Part model, mm, in its own coordinate system. A direction names the side the tool comes from. Give positions to 0.01 mm unless a question says otherwise; leave off trailing zeros. Loops run counter-clockwise (first coordinate to the right, second up) from the corner with the lowest first, then second, coordinate; pieces in that order, holes last. Notation, with made-up numbers: M -9,38 L 47,38 A33 cw 47,74 Z; hole C -12.5,30 d2. An arc over 180 degrees is marked long. Answer in a Markdown table with one row per item.
from build123d import *

# Parameters (mm, degrees)
F1_DEPTH = 4


with BuildPart() as f1:
    # F0 (on Front) → F1 (new body, symmetric)
    with BuildSketch(Plane.XZ):
        with BuildLine():
            ThreePointArc((111.130167, 15.609894), (95.033027, 8.473776), (77.595073, 6.0325))
            Line((77.595073, 6.0325), (-77.595073, 6.0325))
            ThreePointArc((-77.595073, 6.0325), (-95.033027, 8.473776), (-111.130167, 15.609894))
            ThreePointArc((-111.130167, 15.609894), (-161.194556, 29.17665), (-210.450019, 12.91629))
            ThreePointArc((-210.450019, 12.91629), (-213.914336, 11.208725), (-217.731712, 10.621431))
            Line((-217.731712, 10.621431), (-225.425, 10.621431))
            Line((-225.425, 10.621431), (-225.425, 0))
            Line((-225.425, 0), (-225.191568, 0))
            Line((-225.191568, 0), (-217.639167, 0))
            ThreePointArc((-217.639167, 0), (-213.437314, 0.715242), (-209.708742, 2.780405))
            ThreePointArc((-209.708742, 2.780405), (-161.129499, 20.611828), (-111.59344, 5.64248))
            ThreePointArc((-111.59344, 5.64248), (-94.152949, -3.043403), (-74.899881, -6.0325))
            Line((-74.899881, -6.0325), (74.899881, -6.0325))
            ThreePointArc((74.899881, -6.0325), (94.152949, -3.043403), (111.59344, 5.64248))
            ThreePointArc((111.59344, 5.64248), (161.129499, 20.611828), (209.708742, 2.780405))
            ThreePointArc((209.708742, 2.780405), (213.437314, 0.715242), (217.639167, 0))
            Line((217.639167, 0), (225.191568, 0))
            Line((225.191568, 0), (225.425, 0))
            Line((225.425, 0), (225.425, 10.621431))
            Line((225.425, 10.621431), (217.731712, 10.621431))
            ThreePointArc((217.731712, 10.621431), (213.914336, 11.208725), (210.450019, 12.91629))
            ThreePointArc((210.450019, 12.91629), (161.194556, 29.17665), (111.130167, 15.609894))
        make_face()
    extrude(amount=F1_DEPTH, both=True)


solid = f1.part
(1) Which spindle directions (+Z, -Z, +X, -X, +Y, -Y) get a long thin tool onto all of the face, cutting with end or side? Do faces 5 (the face through (-94.795, -0.056, 8.406)), 6 (the face through (221, 0, 0)), 7 (the face through (-222, 0, 0)), 8 (the face through (-213.494, -0.056, 0.696)), 9 (the face through (222, 0, 10.621)). Say none if no direction does.
Recorded:
| item | result |
|---|---|
| face 5 | +Z, +Y, -Y |
| face 6 | -Z, +X, +Y, -Y |
| face 7 | -Z, -X, +Y, -Y |
| face 8 | -Z, +Y, -Y |
| face 9 | +Z, +X, +Y, -Y |
(2) Pull direction X, two halves, no side cores. Call faces 1 (the face through (-1, 0, -6.032)), 2 (the face through (-160.458, -0.056, 29.194)), 3 (the face through (161.931, -0.056, 29.154)), 4 (the face through (225.425, 0, 5)): +X half, -X half, draft (parallel to the pull), parting line (faces both ways), or undercut.
Recorded:
| item | result |
|---|---|
| face 1 | draft |
| face 2 | undercut |
| face 3 | undercut |
| face 4 | +X half |
(3) Drill centre lines: line 1 along Z through (x, y) = (-25, 2); line 2 along X through (y, z) = (0.5, 5.5) (3 decimals); line 3 along X through (y, z) = (-1.5, 21). Where is each one in solid material? Low to high.
Recorded:
| item | result |
|---|---|
| line 1 | z = -6.03 to 6.03 |
| line 2 | x = -225.425 to -206.107, -111.391 to 111.391, 206.107 to 225.425 |
| line 3 | x = -196.34 to -121.16, 121.16 to 196.34 |
(4) Saw through at B-B (x = -12). Write the cut outline in (y, z).
Recorded:
| item | result |
|---|---|
| outline | M -4,-6.03 L 4,-6.03 L 4,6.03 L -4,6.03 Z |
(5) Pin check, flat tips, straight feed: pin 1 Ø1.5 at (y, z) = (0, 19.5) entering from +X; pin 2 Ø2 at (x, y) = (-101.5, 3) entering from -Z; pin 3 Ø2.5 at (x, y) = (-27, 2) entering from +Z. Stop position of each tip, or through.
Recorded:
| item | result |
|---|---|
| pin 1 | stops at x = 200.9 |
| pin 2 | stops at z = -0.64 |
| pin 3 | stops at z = 6.03 |
(6) Saw through at C-C (x = -96). Write the cut outline in (y, z).
Recorded:
| item | result |
|---|---|
| outline | M -4,-2.42 L 4,-2.42 L 4,8.76 L -4,8.76 Z |
